The listing builds one solid part. Answer for the finished solid, in the listing's coordinates (mm). Coordinates: 2 decimals unless noted, no trailing zeros. Loops run counter-clockwise (first coordinate to the right, second up) from the corner with the lowest first, then second, coordinate; pieces in that order, holes last. Notation, with made-up numbers: M 14.5,35 L 23.5,35 A15 ccw 23.5,40 Z; hole C 20.5,8 d9. An arc over 180 degrees is marked long. Answer as a JSON object with one key per item and string values. Group by question number.
1. A straight line is drawn through the part: L1, parallel to Z at x = 0.9, y = 606. Find the intervals that lie inside material, in ascending order.
2. A cutting plane is placed at C-C on z = -304.8. State how many separate pieces and enclosed holes the cut face has, and give its area (3 significant figures).
3. A cutting plane is placed at A-A on y = -609.6. Give the vertices of the cut face in (x, z), and give its area (3 significant figures).
4. A cutting plane is placed at B-B on y = -381. Give the vertices of the cut face in (x, z), and give its area (3 significant figures).
from build123d import *

# Parameters (mm, degrees)
SKETCH1_W           = 914.4
SKETCH1_H           = 1524
BOSS_EXTRUDE1_DEPTH = 2.54
SKETCH3_R           = 25.4
CUT_EXTRUDE1_DEPTH  = 3.54


with BuildPart() as part:
    # Sketch1 → Boss-Extrude1 (new body)
    with BuildSketch(Plane(origin=(0, 0, 0), x_dir=(0, 0, -1), z_dir=(1, 0, 0))):
        Rectangle(SKETCH1_W, SKETCH1_H)
    extrude(amount=BOSS_EXTRUDE1_DEPTH)

    # Sketch3 → Cut-Extrude1 (cut, through all)
    with BuildSketch(Plane.ZY):
        with Locations((-381, -685.8)):
            Circle(SKETCH3_R)
        with Locations((-304.8, -609.6)):
            Circle(SKETCH3_R)
        with Locations((-228.6, -685.8)):
            Circle(SKETCH3_R)
        with Locations((-76.2, -685.8)):
            Circle(SKETCH3_R)
        with Locations((76.2, -685.8)):
            Circle(SKETCH3_R)
        with Locations((228.6, -685.8)):
            Circle(SKETCH3_R)
        with Locations((381, -685.8)):
            Circle(SKETCH3_R)
        with Locations((-228.6, -533.4)):
            Circle(SKETCH3_R)
        with Locations((-76.2, -533.4)):
            Circle(SKETCH3_R)
        with Locations((76.2, -533.4)):
            Circle(SKETCH3_R)
        with Locations((228.6, -533.4)):
            Circle(SKETCH3_R)
        with Locations((381, -533.4)):
            Circle(SKETCH3_R)
        with Locations((-228.6, -381)):
            Circle(SKETCH3_R)
        with Locations((-76.2, -381)):
            Circle(SKETCH3_R)
        with Locations((76.2, -381)):
            Circle(SKETCH3_R)
        with Locations((228.6, -381)):
            Circle(SKETCH3_R)
        with Locations((381, -381)):
            Circle(SKETCH3_R)
        with Locations((-228.6, -228.6)):
            Circle(SKETCH3_R)
        with Locations((-76.2, -228.6)):
            Circle(SKETCH3_R)
        with Locations((76.2, -228.6)):
            Circle(SKETCH3_R)
        with Locations((228.6, -228.6)):
            Circle(SKETCH3_R)
        with Locations((381, -228.6)):
            Circle(SKETCH3_R)
        with Locations((-228.6, -76.2)):
            Circle(SKETCH3_R)
        with Locations((-76.2, -76.2)):
            Circle(SKETCH3_R)
        with Locations((76.2, -76.2)):
            Circle(SKETCH3_R)
        with Locations((228.6, -76.2)):
            Circle(SKETCH3_R)
        with Locations((381, -76.2)):
            Circle(SKETCH3_R)
        with Locations((-228.6, 76.2)):
            Circle(SKETCH3_R)
        with Locations((-76.2, 76.2)):
            Circle(SKETCH3_R)
        with Locations((76.2, 76.2)):
            Circle(SKETCH3_R)
        with Locations((228.6, 76.2)):
            Circle(SKETCH3_R)
        with Locations((381, 76.2)):
            Circle(SKETCH3_R)
        with Locations((-228.6, 228.6)):
            Circle(SKETCH3_R)
        with Locations((-76.2, 228.6)):
            Circle(SKETCH3_R)
        with Locations((76.2, 228.6)):
            Circle(SKETCH3_R)
        with Locations((228.6, 228.6)):
            Circle(SKETCH3_R)
        with Locations((381, 228.6)):
            Circle(SKETCH3_R)
        with Locations((-228.6, 381)):
            Circle(SKETCH3_R)
        with Locations((-76.2, 381)):
            Circle(SKETCH3_R)
        with Locations((76.2, 381)):
            Circle(SKETCH3_R)
        with Locations((228.6, 381)):
            Circle(SKETCH3_R)
        with Locations((381, 381)):
            Circle(SKETCH3_R)
        with Locations((-228.6, 533.4)):
            Circle(SKETCH3_R)
        with Locations((-76.2, 533.4)):
            Circle(SKETCH3_R)
        with Locations((76.2, 533.4)):
            Circle(SKETCH3_R)
        with Locations((228.6, 533.4)):
            Circle(SKETCH3_R)
        with Locations((381, 533.4)):
            Circle(SKETCH3_R)
        with Locations((-228.6, 685.8)):
            Circle(SKETCH3_R)
        with Locations((-76.2, 685.8)):
            Circle(SKETCH3_R)
        with Locations((76.2, 685.8)):
            Circle(SKETCH3_R)
        with Locations((228.6, 685.8)):
            Circle(SKETCH3_R)
        with Locations((381, 685.8)):
            Circle(SKETCH3_R)
        with Locations((-381, -533.4)):
            Circle(SKETCH3_R)
        with Locations((-381, -381)):
            Circle(SKETCH3_R)
        with Locations((-381, -228.6)):
            Circle(SKETCH3_R)
        with Locations((-381, -76.2)):
            Circle(SKETCH3_R)
        with Locations((-381, 76.2)):
            Circle(SKETCH3_R)
        with Locations((-381, 228.6)):
            Circle(SKETCH3_R)
        with Locations((-381, 381)):
            Circle(SKETCH3_R)
        with Locations((-381, 533.4)):
            Circle(SKETCH3_R)
        with Locations((-381, 685.8)):
            Circle(SKETCH3_R)
        with Locations((-152.4, -609.6)):
            Circle(SKETCH3_R)
        with Locations((0, -609.6)):
            Circle(SKETCH3_R)
        with Locations((152.4, -609.6)):
            Circle(SKETCH3_R)
        with Locations((304.8, -609.6)):
            Circle(SKETCH3_R)
        with Locations((-152.4, -457.2)):
            Circle(SKETCH3_R)
        with Locations((0, -457.2)):
            Circle(SKETCH3_R)
        with Locations((152.4, -457.2)):
            Circle(SKETCH3_R)
        with Locations((304.8, -457.2)):
            Circle(SKETCH3_R)
        with Locations((-152.4, -304.8)):
            Circle(SKETCH3_R)
        with Locations((0, -304.8)):
            Circle(SKETCH3_R)
        with Locations((152.4, -304.8)):
            Circle(SKETCH3_R)
        with Locations((304.8, -304.8)):
            Circle(SKETCH3_R)
        with Locations((-152.4, -152.4)):
            Circle(SKETCH3_R)
        with Locations((0, -152.4)):
            Circle(SKETCH3_R)
        with Locations((152.4, -152.4)):
            Circle(SKETCH3_R)
        with Locations((304.8, -152.4)):
            Circle(SKETCH3_R)
        with Locations((-152.4, 0)):
            Circle(SKETCH3_R)
        Circle(SKETCH3_R)
        with Locations((152.4, 0)):
            Circle(SKETCH3_R)
        with Locations((304.8, 0)):
            Circle(SKETCH3_R)
        with Locations((-152.4, 152.4)):
            Circle(SKETCH3_R)
        with Locations((0, 152.4)):
            Circle(SKETCH3_R)
        with Locations((152.4, 152.4)):
            Circle(SKETCH3_R)
        with Locations((304.8, 152.4)):
            Circle(SKETCH3_R)
        with Locations((-152.4, 304.8)):
            Circle(SKETCH3_R)
        with Locations((0, 304.8)):
            Circle(SKETCH3_R)
        with Locations((152.4, 304.8)):
            Circle(SKETCH3_R)
        with Locations((304.8, 304.8)):
            Circle(SKETCH3_R)
        with Locations((-152.4, 457.2)):
            Circle(SKETCH3_R)
        with Locations((0, 457.2)):
            Circle(SKETCH3_R)
        with Locations((152.4, 457.2)):
            Circle(SKETCH3_R)
        with Locations((304.8, 457.2)):
            Circle(SKETCH3_R)
        with Locations((-152.4, 609.6)):
            Circle(SKETCH3_R)
        with Locations((0, 609.6)):
            Circle(SKETCH3_R)
        with Locations((152.4, 609.6)):
            Circle(SKETCH3_R)
        with Locations((304.8, 609.6)):
            Circle(SKETCH3_R)
        with Locations((-304.8, -457.2)):
            Circle(SKETCH3_R)
        with Locations((-304.8, -304.8)):
            Circle(SKETCH3_R)
        with Locations((-304.8, -152.4)):
            Circle(SKETCH3_R)
        with Locations((-304.8, 0)):
            Circle(SKETCH3_R)
        with Locations((-304.8, 152.4)):
            Circle(SKETCH3_R)
        with Locations((-304.8, 304.8)):
            Circle(SKETCH3_R)
        with Locations((-304.8, 457.2)):
            Circle(SKETCH3_R)
        with Locations((-304.8, 609.6)):
            Circle(SKETCH3_R)
    extrude(amount=-CUT_EXTRUDE1_DEPTH, mode=Mode.SUBTRACT)


solid = part.part
From the geometry:
{
 "1": {"L1": "z = -457.2 to -329.94, -279.66 to -177.54, -127.26 to -25.14, 25.14 to 127.26, 177.54 to 279.66, 329.94 to 457.2"},
 "2": {"separate pieces": "10", "enclosed holes": "0", "area": "2,710 mm²"},
 "3": {"outline": "M 0,-457.2 L 2.54,-457.2 L 2.54,-330.2 L 0,-330.2 Z; M 0,-279.4 L 2.54,-279.4 L 2.54,-177.8 L 0,-177.8 Z; M 0,-127 L 2.54,-127 L 2.54,-25.4 L 0,-25.4 Z; M 0,25.4 L 2.54,25.4 L 2.54,127 L 0,127 Z; M 0,177.8 L 2.54,177.8 L 2.54,279.4 L 0,279.4 Z; M 0,330.2 L 2.54,330.2 L 2.54,457.2 L 0,457.2 Z", "area": "1,680 mm²"},
 "4": {"outline": "M 0,-457.2 L 2.54,-457.2 L 2.54,-406.4 L 0,-406.4 Z; M 0,-355.6 L 2.54,-355.6 L 2.54,-254 L 0,-254 Z; M 0,-203.2 L 2.54,-203.2 L 2.54,-101.6 L 0,-101.6 Z; M 0,-50.8 L 2.54,-50.8 L 2.54,50.8 L 0,50.8 Z; M 0,101.6 L 2.54,101.6 L 2.54,203.2 L 0,203.2 Z; M 0,254 L 2.54,254 L 2.54,355.6 L 0,355.6 Z; M 0,406.4 L 2.54,406.4 L 2.54,457.2 L 0,457.2 Z", "area": "1,550 mm²"}
}
